Check sheet for the modelled part. Datum: model origin and axes. Units: mm. A direction names the side the tool comes from. Give positions to 0.01 mm unless a question says otherwise; leave off trailing zeros. Order: outer loops, then holes, each group sorted by start corner. A loop starts at its lowest first (then second) coordinate and runs counter-clockwise, first axis right, second up.
```python
from build123d import *

# Parameters (mm, degrees)
SKETCH1_R           = 1.6
BOSS_EXTRUDE1_DEPTH = 2.5
FILLET1_R           = 2
SKETCH2_R           = 3.4
CUT_EXTRUDE1_DEPTH  = 3.5000001


with BuildPart() as part:
    # Sketch1 → Boss-Extrude1 (new body)
    with BuildSketch(Plane(origin=(0, 0, 0), x_dir=(0, 0, -1), z_dir=(1, 0, 0))):
        with BuildLine():
            ThreePointArc((-34.4875, 20.263571841), (-19, 0), (-34.4875, -20.263571841))
            ThreePointArc((-34.4875, -20.263571841), (40, 0), (-34.4875, 20.263571841))
        make_face()
        with BuildLine():
            Line((-9.682458366, 2.5), (-14.120471411, 2.5))
            ThreePointArc((-14.120471411, 2.5), (-18.092232837, 14.001776242), (-26.8625, 22.436713078))
            ThreePointArc((-26.8625, 22.436713078), (-15.727733284, 31.267209753), (-2, 34.942810419))
            Line((-2, 34.942810419), (-2, 9.797958971))
            ThreePointArc((-2, 9.797958971), (-6.887307867, 7.250171746), (-9.682458366, 2.5))
        make_face(mode=Mode.SUBTRACT)
        with BuildLine():
            Line((-14.120471411, -2.5), (-9.682458366, -2.5))
            ThreePointArc((-9.682458366, -2.5), (-6.887307867, -7.250171746), (-2, -9.797958971))
            Line((-2, -9.797958971), (-2, -34.942810419))
            ThreePointArc((-2, -34.942810419), (-15.727733284, -31.267209753), (-26.8625, -22.436713078))
            ThreePointArc((-26.8625, -22.436713078), (-18.092232837, -14.001776242), (-14.120471411, -2.5))
        make_face(mode=Mode.SUBTRACT)
        with BuildLine():
            ThreePointArc((2, -9.797958971), (6.887307867, -7.250171746), (9.682458366, -2.5))
            Line((9.682458366, -2.5), (34.910600109, -2.5))
            ThreePointArc((34.910600109, -2.5), (24.570960239, -24.925246497), (2, -34.942810419))
            Line((2, -34.942810419), (2, -9.797958971))
        make_face(mode=Mode.SUBTRACT)
        with BuildLine():
            Line((34.910600109, 2.5), (9.682458366, 2.5))
            ThreePointArc((9.682458366, 2.5), (6.887307867, 7.250171746), (2, 9.797958971))
            Line((2, 9.797958971), (2, 34.942810419))
            ThreePointArc((2, 34.942810419), (24.570960239, 24.925246497), (34.910600109, 2.5))
        make_face(mode=Mode.SUBTRACT)
        Circle(SKETCH1_R, mode=Mode.SUBTRACT)
    extrude(amount=BOSS_EXTRUDE1_DEPTH)

    # Fillet1
    fillet1_edges = [part.edges().sort_by_distance(p)[0] for p in [
        (1.25, 20.263571841, 34.4875),
        (1.25, -20.263571841, 34.4875),
        (1.25, 9.797958971, 2),
        (1.25, 34.942810419, 2),
        (1.25, 22.436713078, 26.8625),
        (1.25, 2.5, 9.682458366),
        (1.25, 2.5, -34.910600109),
        (1.25, 34.942810419, -2),
        (1.25, 9.797958971, -2),
        (1.25, 2.5, -9.682458366),
        (1.25, -22.436713078, 26.8625),
        (1.25, -34.942810419, 2),
        (1.25, -9.797958971, 2),
        (1.25, -2.5, 9.682458366),
        (1.25, -9.797958971, -2),
        (1.25, -34.942810419, -2),
        (1.25, -2.5, -34.910600109),
        (1.25, -2.5, -9.682458366),
    ]]
    fillet(fillet1_edges, radius=FILLET1_R)

    # Sketch2 → Cut-Extrude1 (cut, through all)
    with BuildSketch(Plane.ZY):
        Circle(SKETCH2_R)
    extrude(amount=-CUT_EXTRUDE1_DEPTH, mode=Mode.SUBTRACT)


solid = part.part
```
(1) Sectioned sample at B-B (z = 6). Enter the section's corners in (x, y), plus the area to 3 significant figures.
(2) Sectioned sample at C-C (y = -16). Enter the section's corners in (x, z).
(3) Thickness scan on L1, parallel to Z at x = 0.3, y = 3.5; L2, parallel to Z at x = 1.3, y = 14; L3, parallel to Y at x = 0.5, z = -6.5. Record the ranges inside material, lowest first.
(4) Tool access check on faces 1 (the face through (1, 2.5, 13)), 2 (the face through (2.5, -3, -3)). Record the directions out of +Z, -Z, +X, -X, +Y, -Y that give a thin tool (end or side, any length) a straight path to the whole face; none if there is none.
(5) Sectioned sample at A-A (y = 0). Enter the section's corners in (x, z), plus the area to 4 significant figures.
(6) Go/stop test with flat-tipped pins: P1, Ø0.8, axis at x = 1, z = 13, coming from the -Y side; P2, Ø1.5, axis at x = 1.5, y = -8.5, coming from the -Z side; P3, Ø1.2, axis at x = 1.5, y = -27.5, coming from the -Z side. Record where each tip stops, or that it passes through.
(7) Sectioned sample at D-D (x = 1.5). Count the separate pieces of the cut face and the enclosed holes in it, plus the area to 3 significant figures.
Values follow:
1. outline: (0, -39.55) - (2.5, -39.55) - (2.5, -34.48) - (0, -34.48) - close; (0, -8) - (2.5, -8) - (2.5, 8) - (0, 8) - close; (0, 34.48) - (2.5, 34.48) - (2.5, 39.55) - (0, 39.55) - close
1. area: 65.3 mm2
2. outline: (0, -36.66) - (2.5, -36.66) - (2.5, -31.13) - (0, -31.13) - close; (0, -2) - (2.5, -2) - (2.5, 2) - (0, 2) - close; (0, 19.51) - (2.5, 19.51) - (2.5, 26.4) - (0, 26.4) - close
3. L1: z = -39.85 to -34.42, -9.39 to 9.39, 14.24 to 19.29
3. L2: z = -37.47 to -32.08, -2 to 2, 18.09 to 24.35
3. L3: y = -39.47 to -34.39, -7.6 to 7.6, 34.39 to 39.47
4. face 1: +X, -X
4. face 2: +Z, -Z, +X, +Y, -Y
5. outline: (0, -40) - (2.5, -40) - (2.5, -3.4) - (0, -3.4) - close; (0, 3.4) - (2.5, 3.4) - (2.5, 19) - (0, 19) - close
5. area: 130.5 mm2
6. P1: stops at y = -37.96
6. P2: stops at z = -39.24
6. P3: stops at z = -29.6
7. separate pieces: 1
7. enclosed holes: 5
7. area: 1,860 mm2
